Check sheet for the modelled part. Datum: model origin and axes. Units: mm. Coordinates: 2 decimals unless noted, no trailing zeros. Loops run counter-clockwise (first coordinate to the right, second up) from the corner with the lowest first, then second, coordinate; pieces in that order, holes last.
```python
from build123d import *

# Parameters (mm, degrees)
F1_DEPTH = 20
F3_DEPTH = 25
F5_D     = 2.7


with BuildPart() as f1:
    # F0 (on Front) → F1 (new body)
    with BuildSketch(Plane.XZ):
        Polygon((-34.35, 0), (-6.35, 0), (-28.11456562, 21.76456562), (-24.579031714, 25.3000995259), (-34.35, 25.3000995259), align=None)
    extrude(amount=F1_DEPTH)

    # F2 (on face) → F3 (join)
    with BuildSketch(Plane.XZ):
        Polygon((-34.35, 25.3000995259), (-34.35, 0), (0, 0), (0, 10), (-14.3736449024, 25.3000995259), (-24.579031714, 25.3000995259), align=None)
    extrude(amount=-F3_DEPTH)

    # F5 (through all)
    with Locations(Plane(origin=(-3.175, 0, -3.175), x_dir=(0.7071067812, 0, -0.7071067812), z_dir=(0.7071067812, 0, 0.7071067812))):
        with Locations((-20.2698719395, -15)):
            Hole(F5_D / 2)


solid = f1.part
```
1) Depth check by flat-ended pin: pin 1 (5 mm diameter, centred on x = -13.5, z = 13, fed in from -Y); pin 2 (1.5 mm diameter, centred on x = -13, y = -12, fed in from +Z). Enter the tip coordinate at first touch or a pass-through.
Answer sheet:
pin 1: stops at y = 0
pin 2: stops at z = 7.4
2) Scan lines: line 1 (Y direction, x = -4, z = 2.25); line 2 (X direction, y = 10.5, z = 16.75); line 3 (Z direction, x = -26.5, y = -1.5). Record each from-to range of solid material in increasing order.
Answer sheet:
line 1: y = 0 to 25
line 2: x = -34.35 to -6.34
line 3: z = 0 to 20.15, 23.38 to 25.3
3) Mould release check, pull along Z, two halves, no side actions. Record for faces 1 (the flat face through (-26.37, -9.86, 23.51)), 2 (the flat face through (-17, 2, 0)), 3 (the cylindrical face through (-24.56, -14.594, 5.927)), 4 (the flat face through (0, 12, 5)): +Z half, -Z half, draft (parallel to the pull), parting line (faces both ways), or undercut.
Answer sheet:
face 1: undercut
face 2: -Z half
face 3: undercut
face 4: draft
4) Section check D-D on x = -11. Enter the section's corners in (y, z).
Answer sheet:
outline: (-20, 0) - (25, 0) - (25, 21.71) - (0, 21.71) - (0, 4.65) - (-20, 4.65) - close
5) Section check B-B on y = 7. Enter the section's corners in (x, z).
Answer sheet:
outline: (-34.35, 0) - (0, 0) - (0, 10) - (-14.37, 25.3) - (-34.35, 25.3) - close
6) Section check C-C on z = 15.5. Enter the section's corners in (x, y).
Answer sheet:
outline: (-34.35, -20) - (-21.85, -20) - (-21.85, 0) - (-5.17, 0) - (-5.17, 25) - (-34.35, 25) - close
7) Section check A-A on y = -14.5. Enter the section's corners in (x, z), plus the area to 3 significant figures.
Answer sheet:
outline: (-34.35, 0) - (-30.44, 0) - (-18.39, 12.04) - (-28.11, 21.76) - (-24.58, 25.3) - (-34.35, 25.3) - close; (-26.89, 0) - (-6.35, 0) - (-16.62, 10.27) - close
area: 361 mm2
